Check sheet for the modelled part. Datum: model origin and axes. Units: mm. A direction names the side the tool comes from. Give positions to 0.01 mm unless a question says otherwise; leave off trailing zeros. Loops run counter-clockwise (first coordinate to the right, second up) from the corner with the lowest first, then second, coordinate; pieces in that order, holes last.
```python
from build123d import *

# Parameters (mm, degrees)
SCHIZZO1_R                   = 12.5
SCHIZZO1_R_2                 = 2.55
ESTRUSIONE_ESTRUSIONE1_DEPTH = 3


with BuildPart() as part:
    # Schizzo1 → Estrusione-Estrusione1 (new body)
    with BuildSketch(Plane.XY):
        with BuildLine():
            Line((-15.75, -41), (15.75, -41))
            ThreePointArc((15.75, -41), (18.578427125, -39.828427125), (19.75, -37))
            Line((19.75, -37), (19.75, 37))
            ThreePointArc((19.75, 37), (18.578427125, 39.828427125), (15.75, 41))
            Line((15.75, 41), (-15.75, 41))
            ThreePointArc((-15.75, 41), (-18.578427125, 39.828427125), (-19.75, 37))
            Line((-19.75, 37), (-19.75, -37))
            ThreePointArc((-19.75, -37), (-18.578427125, -39.828427125), (-15.75, -41))
        make_face()
        with Locations((0, 19.75)):
            Circle(SCHIZZO1_R, mode=Mode.SUBTRACT)
        with Locations((-10, -12.8)):
            Circle(SCHIZZO1_R_2, mode=Mode.SUBTRACT)
        with Locations((0, -12.8)):
            Circle(SCHIZZO1_R_2, mode=Mode.SUBTRACT)
        with Locations((10, -12.8)):
            Circle(SCHIZZO1_R_2, mode=Mode.SUBTRACT)
        with Locations((10, -32.8)):
            Circle(SCHIZZO1_R_2, mode=Mode.SUBTRACT)
        with Locations((0, -32.8)):
            Circle(SCHIZZO1_R_2, mode=Mode.SUBTRACT)
        with Locations((-10, -32.8)):
            Circle(SCHIZZO1_R_2, mode=Mode.SUBTRACT)
        with BuildLine():
            Line((-14.309257017, 36.242285819), (-11.809257017, 33.242285819))
            ThreePointArc((-11.809257017, 33.242285819), (-12.007714181, 31.059257017), (-14.190742983, 31.257714181))
            Line((-14.190742983, 31.257714181), (-16.690742983, 34.257714181))
            ThreePointArc((-16.690742983, 34.257714181), (-16.492285819, 36.440742983), (-14.309257017, 36.242285819))
        make_face(mode=Mode.SUBTRACT)
        with BuildLine():
            Line((14.309257017, 36.242285819), (11.809257017, 33.242285819))
            ThreePointArc((11.809257017, 33.242285819), (12.007714181, 31.059257017), (14.190742983, 31.257714181))
            Line((14.190742983, 31.257714181), (16.690742983, 34.257714181))
            ThreePointArc((16.690742983, 34.257714181), (16.492285819, 36.440742983), (14.309257017, 36.242285819))
        make_face(mode=Mode.SUBTRACT)
        with BuildLine():
            Line((-11.903984489, 5.653984489), (-14.403984489, 3.153984489))
            ThreePointArc((-14.403984489, 3.153984489), (-16.596015511, 3.153984489), (-16.596015511, 5.346015511))
            Line((-16.596015511, 5.346015511), (-14.096015511, 7.846015511))
            ThreePointArc((-14.096015511, 7.846015511), (-11.903984489, 7.846015511), (-11.903984489, 5.653984489))
        make_face(mode=Mode.SUBTRACT)
        with BuildLine():
            Line((11.903984489, 5.653984489), (14.403984489, 3.153984489))
            ThreePointArc((14.403984489, 3.153984489), (16.596015511, 3.153984489), (16.596015511, 5.346015511))
            Line((16.596015511, 5.346015511), (14.096015511, 7.846015511))
            ThreePointArc((14.096015511, 7.846015511), (11.903984489, 7.846015511), (11.903984489, 5.653984489))
        make_face(mode=Mode.SUBTRACT)
    extrude(amount=ESTRUSIONE_ESTRUSIONE1_DEPTH)


solid = part.part
```
(1) Release check for a two-part mould opening along X. For faces 1 (the face through (0, 1, 0)), 2 (the face through (-18.609, -39.797, 1.479)), 3 (the face through (-15.36, 6.58, 1.48)) record: pulls with the +X half, pulls with the -X half, needs draft (parallel to the pull), parting line crosses it, or undercut.
(2) Section check A-A on y = -12.8. Record the boundary of the cut face in (x, z), plus the area to 3 significant figures.
(3) Gauge pin test, flat ends, axial feed: pin 1 Ø6 at (x, y) = (0, -32.8) entering from -Z; pin 2 Ø20 at (x, y) = (0, 19.75) entering from +Z. Record the tip position at first contact, or that the pin passes through.
(4) Section check D-D on y = 19.75. Record the boundary of the cut face in (x, z).
(5) Section check C-C on z = 2.5. Give the number of separate pieces and of enclosed holes in the cut face, plus the area to 3 significant figures.
(6) Material ranges on line 1 (Y direction, x = 0, z = 2.35); line 2 (Y direction, x = 10, z = 2.4); line 3 (X direction, y = -33.5, z = 0.55), recorded low to high.
(7) Access from +Z, -Z, +X, -X, +Y, -Y to the whole of each face (thin tool, end or side, straight path). Record for faces 4 (the face through (-15.423, 32.737, 1.479)), 5 (the face through (0, 1, 3)).
(8) Section check B-B on x = -10. Record the boundary of the cut face in (y, z).
Computed values:
1. face 1: needs draft
1. face 2: pulls with the -X half
1. face 3: undercut
2. outline: (-19.75, 0) - (-12.55, 0) - (-12.55, 3) - (-19.75, 3) - close; (-7.45, 0) - (-2.55, 0) - (-2.55, 3) - (-7.45, 3) - close; (2.55, 0) - (7.45, 0) - (7.45, 3) - (2.55, 3) - close; (12.55, 0) - (19.75, 0) - (19.75, 3) - (12.55, 3) - close
2. area: 72.6 mm2
3. pin 1: stops at z = 0
3. pin 2: passes through
4. outline: (-19.75, 0) - (-12.5, 0) - (-12.5, 3) - (-19.75, 3) - close; (12.5, 0) - (19.75, 0) - (19.75, 3) - (12.5, 3) - close
5. separate pieces: 1
5. enclosed holes: 11
5. area: 2,540 mm2
6. line 1: y = -41 to -35.35, -30.25 to -15.35, -10.25 to 7.25, 32.25 to 41
6. line 2: y = -41 to -35.35, -30.25 to -15.35, -10.25 to 12.25, 27.25 to 41
6. line 3: x = -19.75 to -12.45, -7.55 to -2.45, 2.45 to 7.55, 12.45 to 19.75
7. face 4: +Z, -Z
7. face 5: +Z, +X, -X, +Y, -Y
8. outline: (-41, 0) - (-35.35, 0) - (-35.35, 3) - (-41, 3) - close; (-30.25, 0) - (-15.35, 0) - (-15.35, 3) - (-30.25, 3) - close; (-10.25, 0) - (12.25, 0) - (12.25, 3) - (-10.25, 3) - close; (27.25, 0) - (41, 0) - (41, 3) - (27.25, 3) - close
